Input: dimensioned drawing with shaded views. Units: mm. Origin: part minimum x, y, z. Coordinates: 2 decimals unless noted, no trailing zeros. Loops run counter-clockwise (first coordinate to the right, second up) from the corner with the lowest first, then second, coordinate; pieces in that order, holes last.
Item 1: Ray query, line 1 along Y through (x, z) = (15, 8.75); line 2 along Z through (x, y) = (13, 27.5); line 3 along Y through (x, z) = (16.5, 11.75). Return the intervals inside material, ascending.
Item 2: Section D-D on z = 15.5. Return loops of the section in (x, y).
Item 3: Section A-A on x = 15. Return loops of the section in (y, z).
Item 4: Contact query for flat-ended pins moving along their axis: P1, Ø5, axis at y = 8.5, z = 12, coming from the +X side; P2, Ø3, axis at y = 20, z = 2, coming from the -X side; P3, Ø2, axis at y = 23, z = 6.5, coming from the -X side; P4, Ø1, axis at x = 24.5, y = 6, coming from the +Z side. Output: stop coordinate, or through.
Item 5: Section C-C on z = 6.5. Return loops of the section in (x, y).
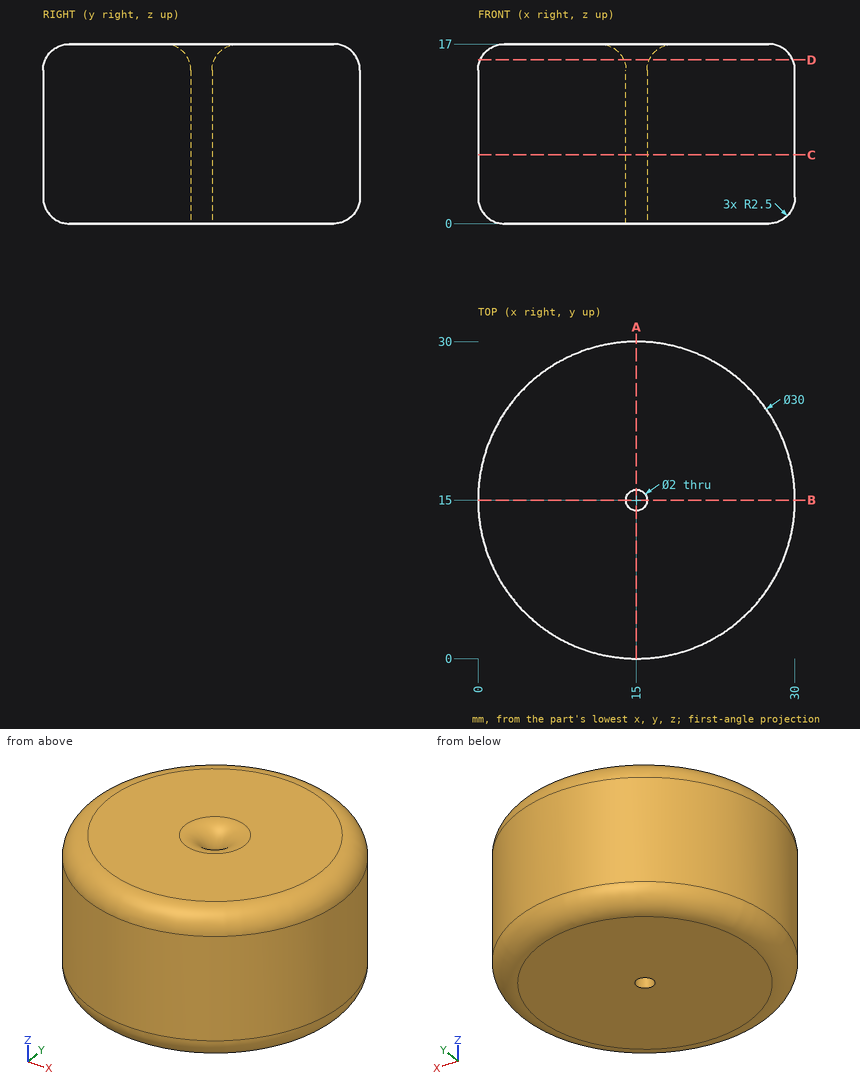
Results found:
1. line 1: y = 0 to 14, 16 to 30
1. line 2: z = 0.01 to 16.99
1. line 3: y = 0.08 to 29.92
2. outline: circle Ø29.58 at (15, 15); hole circle Ø2.42 at (15, 15)
3. outline: (0, 2.5) arc R2.5 ccw to (2.5, 0) - (14, 0) - (14, 14.5) arc R2.5 ccw to (11.5, 17) - (2.5, 17) arc R2.5 ccw to (0, 14.5) - close; (16, 0) - (27.5, 0) arc R2.5 ccw to (30, 2.5) - (30, 14.5) arc R2.5 ccw to (27.5, 17) - (18.5, 17) arc R2.5 ccw to (16, 14.5) - close
4. P1: stops at x = 29.46
4. P2: stops at x = 0.43
4. P3: stops at x = 1.73
4. P4: stops at z = 17
5. outline: circle Ø30 at (15, 15); hole circle Ø2 at (15, 15)
